Design review of the part built by this model. Coordinates are the model's own, in mm. Coordinates: 2 decimals unless noted, no trailing zeros. Order: outer loops, then holes, each group sorted by start corner. A loop starts at its lowest first (then second) coordinate and runs counter-clockwise, first axis right, second up. Notation, with made-up numbers: (-18, 33) -> (30, 33) arc R32 ccw to (30, 59) -> close; hole circle Ø3 at (8, -35.75). An arc over 180 degrees is marked (long way). Use a Markdown table: item, result. Add a question column.
Q1. Add section C-C (x = 631.5). State the section outline as (y, z) points, then the cut area to 3 significant figures.
Q2. Add section A-A (z = -25.4). State the section outline as (x, y) points, then the cut area to 3 significant figures.
Q3. The part is to be moulded in two halves that separate along Z. For faces 1 (the face through (1231.077, 260.1, -44.1)), 2 (the face through (813.164, 253.062, -16.304)), 3 (the face through (808.599, 251.537, -35.128)), say which applies: pulls with the +Z half, pulls with the -Z half, needs draft (parallel to the pull), parting line crosses it, or undercut.
Q4. Wall thickness on probe 1 along Y at (x, z) = (935, -25.4); probe 2 along Z at (x, y) = (779.5, 273); probe 3 along Z at (x, y) = (1000.5, 276.5): over which ranges is each line inside the solid? List them lowest first.
Q5. Add section B-B (y = 275). State the section outline as (x, z) points, then the cut area to 3 significant figures.
Q6. Insertion check: pin 1 (2 mm diameter, centred on x = 1127, z = -34.5, fed in from -Y); pin 2 (2 mm diameter, centred on x = 873.5, y = 288.5, fed in from +Z); pin 3 (1 mm diameter, centred on x = 518, y = 291.5, fed in from +Z). Each pin has a flat end and moves straight along its axis. Give the tip position at first contact, or say it passes through.
from build123d import *

# Parameters (mm, degrees)
SKETCH004_R          = 25.4
PAD002_DEPTH         = 833.289565
SKETCH013_R          = 23.749
POCKET004_DEPTH      = 833.290565
SKETCH012_R          = 25.4
POCKET005_DEPTH      = 0.001
POCKET005_DEPTH_BACK = 300.401


with BuildPart() as cargo_side_tube_r:
    # Sketch004 → Pad002 (new body)
    with BuildSketch(Plane.YZ):
        with Locations((-275, -25.4)):
            Circle(SKETCH004_R)
    extrude(amount=PAD002_DEPTH)

    # Sketch013 (on Face2 of Pad002) → Pocket004 (cut, through all)
    with BuildSketch(Plane(origin=(0, 0, 0), x_dir=(0, 1, 0), z_dir=(-1, 0, 0))):
        with Locations((-275, 25.4)):
            Circle(SKETCH013_R)
    extrude(amount=-POCKET004_DEPTH, mode=Mode.SUBTRACT)

    # Sketch012 → Pocket005 (cut, two sides)
    with BuildSketch(Plane.XZ) as pocket005_sk:
        with Locations((0, -25.4)):
            Circle(SKETCH012_R)
    extrude(amount=-POCKET005_DEPTH, mode=Mode.SUBTRACT)
    extrude(pocket005_sk.sketch, amount=POCKET005_DEPTH_BACK, mode=Mode.SUBTRACT)


with BuildPart() as cargo_side_tube_r_1:
    # Body002 placement: moved
    add(cargo_side_tube_r.part.moved(Location((397.787357, 0, 0))))


with BuildPart() as cargo_side_tube_l:
    # Part__Mirroring: instance of cargo_side_tube_r
    add(cargo_side_tube_r_1.part.mirror(Plane(origin=(0, 0, 0), x_dir=(1, 0, 0), z_dir=(0, 1, 0))))


solid = cargo_side_tube_l.part
Established:
| question | item | result |
|---|---|---|
| 1 | outline | circle Ø50.8 at (275, -25.4); hole circle Ø47.5 at (275, -25.4) |
| 1 | area | 255 mm^2 |
| 2 | outline | (423.19, 249.6) -> (1231.08, 249.6) -> (1231.08, 251.25) -> (423.19, 251.25) -> close; (423.19, 298.75) -> (1231.08, 298.75) -> (1231.08, 300.4) -> (423.19, 300.4) -> close |
| 2 | area | 2,670 mm^2 |
| 3 | face 1 | needs draft |
| 3 | face 2 | undercut |
| 3 | face 3 | parting line crosses it |
| 4 | probe 1 | 249.6 to 251.25, 298.75 to 300.4 |
| 4 | probe 2 | -50.72 to -49.06, -1.74 to -0.08 |
| 4 | probe 3 | -50.76 to -49.1, -1.7 to -0.04 |
| 5 | outline | (397.79, -50.8) -> (1231.08, -50.8) -> (1231.08, -49.15) -> (406.8, -49.15) arc R25.4 cw to start; (397.79, 0) arc R25.4 cw to (406.8, -1.65) -> (1231.08, -1.65) -> (1231.08, 0) -> close |
| 5 | area | 2,730 mm^2 |
| 6 | pin 1 | y = 250.93 |
| 6 | pin 2 | z = -3.29 |
| 6 | pin 3 | z = -5.67 |
